Answer from the drawing. Dimensions are ordinates in mm from the lowest x, y and z of the part. Give positions to 0.01 mm unless a question says otherwise; leave off trailing zeros. Write each loop counter-clockwise with the first axis right and the second up, starting at its lowest first coordinate (ties: lowest second). Pieces come first, ordered by that corner, then holes. Notation, with made-up numbers: (47.25, -20) - (59.25, -20) arc R32 ccw to (59.25, 18) - close; hole circle Ø10 at (10, 0). An arc over 180 degrees is marked (long way). Answer as a JSON object with one key per item and string values. Group by question number.
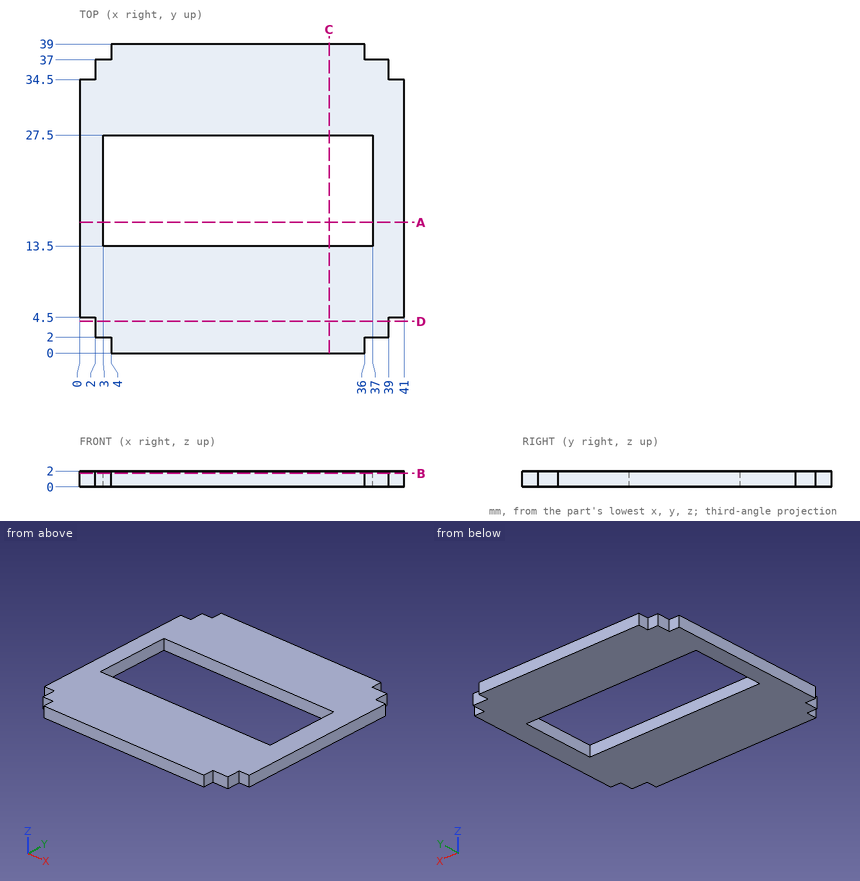
1) Find section A-A, the plane y = 16.5. Write down the section's boundary in (x, z), and give its area (3 significant figures).
2) Find section B-B, the plane z = 1.7. Write down the section's boundary in (x, y).
3) Find the intervals of material crossed by line 1 (Y direction, x = 25.5, z = 0.25); line 2 (X direction, y = 15, z = 0.45); line 3 (Y direction, x = 3.5, z = 0.25), in increasing order. Write a range as [from, to].
4) Find section D-D, the plane y = 4. Write down the section's boundary in (x, z).
5) Find section C-C, the plane x = 31.5. Write down the section's boundary in (y, z), and give its area (3 significant figures).
6) Flat-ended cylindrical pins translate along their axes: pin 1 Ø6 at (x, y) = (13.5, 27) entering from -Z; pin 2 Ø1 at (y, z) = (38, 1.5) entering from -X; pin 3 Ø1 at (x, z) = (40, 1) entering from -Y; pin 4 Ø1 at (x, z) = (38, 1.5) entering from -Y. Find the tip coordinate at first contact, or state that the pin passes through.
Values follow:
{
 "1": {"outline": "(0, 0) - (3, 0) - (3, 2) - (0, 2) - close; (37, 0) - (41, 0) - (41, 2) - (37, 2) - close", "area": "14.0 mm2"},
 "2": {"outline": "(0, 4.5) - (2, 4.5) - (2, 2) - (4, 2) - (4, 0) - (36, 0) - (36, 2) - (39, 2) - (39, 4.5) - (41, 4.5) - (41, 34.5) - (39, 34.5) - (39, 37) - (36, 37) - (36, 39) - (4, 39) - (4, 37) - (2, 37) - (2, 34.5) - (0, 34.5) - close; hole (3, 13.5) - (37, 13.5) - (37, 27.5) - (3, 27.5) - close"},
 "3": {"line 1": "y = [0, 13.5], [27.5, 39]", "line 2": "x = [0, 3], [37, 41]", "line 3": "y = [2, 13.5], [27.5, 37]"},
 "4": {"outline": "(2, 0) - (39, 0) - (39, 2) - (2, 2) - close"},
 "5": {"outline": "(0, 0) - (13.5, 0) - (13.5, 2) - (0, 2) - close; (27.5, 0) - (39, 0) - (39, 2) - (27.5, 2) - close", "area": "50.0 mm2"},
 "6": {"pin 1": "stops at z = 0", "pin 2": "stops at x = 4", "pin 3": "stops at y = 4.5", "pin 4": "stops at y = 2"}
}
